```python
from build123d import *

# Parameters (mm, degrees)
F0_W      = 101.6
F0_H      = 63.5
F1_DEPTH  = 6.35
F2_W      = 101.6
F2_H      = 6.35
F3_DEPTH  = 6.35
F4_W      = 101.6
F4_H      = 20.32
F5_DEPTH  = 6.35
F6_W      = 101.6
F6_H      = 8.8265
F7_DEPTH  = 6.35
F8_W      = 12.7
F8_H      = 6.35
F9_DEPTH  = 6.35
F10_W     = 12.7
F10_H     = 6.35
F11_DEPTH = 6.35
F12_W     = 101.6
F12_H     = 6.9977
F13_DEPTH = 6.35
F14_W     = 12.7
F14_H     = 6.35
F15_DEPTH = 6.35
F16_W     = 12.7
F16_H     = 6.35
F17_DEPTH = 6.35
F19_DEPTH = 6.35


with BuildPart() as f1:
    # F0 (on Top) → F1 (new body)
    with BuildSketch(Plane.XY):
        Rectangle(F0_W, F0_H)
    extrude(amount=F1_DEPTH)

    # F2 (on face) → F3 (join)
    with BuildSketch(Plane.XY.offset(6.35)):
        with Locations((0, -28.575)):
            Rectangle(F2_W, F2_H)
    extrude(amount=F3_DEPTH)

    # F4 (on face) → F5 (join)
    with BuildSketch(Plane.XY.offset(6.35)):
        with Locations((0, 3.937)):
            Rectangle(F4_W, F4_H)
    extrude(amount=F5_DEPTH)

    # F6 (on face) → F7 (join)
    with BuildSketch(Plane.XY.offset(6.35)):
        with Locations((0, 27.33675)):
            Rectangle(F6_W, F6_H)
    extrude(amount=F7_DEPTH)

    # F8 (on face) → F9 (join)
    with BuildSketch(Plane.XZ.offset(31.75)):
        with Locations((-44.45, 3.175)):
            Rectangle(F8_W, F8_H)
        with Locations((-19.05, 3.175)):
            Rectangle(F8_W, F8_H)
        with Locations((6.35, 3.175)):
            Rectangle(F8_W, F8_H)
        with Locations((31.75, 3.175)):
            Rectangle(F8_W, F8_H)
    extrude(amount=F9_DEPTH)

    # F10 (on face) → F11 (join)
    with BuildSketch(Plane(origin=(0, 31.75, 0), x_dir=(-1, 0, 0), z_dir=(0, 1, 0))):
        with Locations((-44.45, 3.175)):
            Rectangle(F10_W, F10_H)
        with Locations((-19.05, 3.175)):
            Rectangle(F10_W, F10_H)
        with Locations((6.35, 3.175)):
            Rectangle(F10_W, F10_H)
        with Locations((31.75, 3.175)):
            Rectangle(F10_W, F10_H)
    extrude(amount=F11_DEPTH)

    # F12 (on face) → F13 (join)
    with BuildSketch(Plane.XY.offset(6.35)):
        with Locations((0, 19.42465)):
            Rectangle(F12_W, F12_H)
    extrude(amount=F13_DEPTH)

    # F14 (on face) → F15 (join)
    with BuildSketch(Plane.YZ.offset(50.8)):
        Polygon((-19.05, 0), (-19.05, 6.35), (-25.4, 6.35), (-31.75, 6.35), (-31.75, 0), align=None)
        Polygon((6.35, 6.35), (0, 6.35), (-6.223, 6.35), (-6.35, 6.35), (-6.35, 0), (6.35, 0), align=None)
        with Locations((25.4, 3.175)):
            Rectangle(F14_W, F14_H)
    extrude(amount=F15_DEPTH)

    # F16 (on face) → F17 (join)
    with BuildSketch(Plane(origin=(-50.8, 0, 0), x_dir=(0, -1, 0), z_dir=(-1, 0, 0))):
        with Locations((-25.4, 3.175)):
            Rectangle(F16_W, F16_H)
        Polygon((6.223, 6.35), (0, 6.35), (-6.35, 6.35), (-6.35, 0), (6.35, 0), (6.35, 6.35), align=None)
        Polygon((25.4, 6.35), (19.05, 6.35), (19.05, 0), (31.75, 0), (31.75, 6.35), align=None)
    extrude(amount=F17_DEPTH)

    # F18 (on face) → F19 (join)
    with BuildSketch(Plane.XY.offset(6.35)):
        Polygon((50.8, -6.223), (-50.8, -6.223), (-50.8, -6.35), (-50.8, -19.05), (50.8, -19.05), (50.8, -6.35), align=None)
    extrude(amount=F19_DEPTH)


solid = f1.part
```
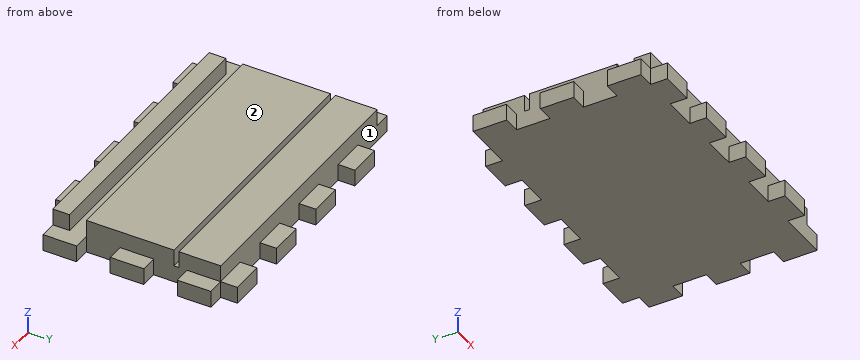
Can you work these out from the model? Positions are in its coordinate system, mm. Face numbers are marked on the shaded views. Round coordinates to 2 decimals unless told otherwise and drop trailing zeros. Loops run counter-clockwise (first coordinate to the right, second up) from the corner with the lowest first, then second, coordinate; pieces in that order, holes last. Notation, with made-up numbers: (72, 88) -> (96, 88) arc R15 cw to (96, 97) -> close; hole circle Ø1 at (-16.75, -32). An arc over 180 degrees is marked (long way). One line per item, written item: value. Start each with the question number.
1. If we section it at C-C, the plane x = -39.5: Write out the boundary of the cut face in (y, z).
2. If we mould it in two halves opening along X, with no side actions, what happens to the marked faces 1 and 2? For each: pulls with the +X half, pulls with the -X half, needs draft (parallel to the pull), parting line crosses it, or undercut.
3. If we section it at A-A, the plane z = 10.75: Write out the boundary of the cut face in (x, y), then the cut area to 3 significant figures.
4. If I drill on probe 1 along Y at (x, z) = (-2.5, 9.5); probe 2 along X at (y, z) = (7, 8.25); probe 3 along Y at (x, z) = (-9.5, 4.25), over which ranges is the centre line in solid material (lowest first)?
5. If we section it at B-B, the plane y = 5: Write out the boundary of the cut face in (x, z).
6. For pin 1 (3 mm diameter, centred on x = 14, z = 10.5, fed in from -Y); pin 2 (5 mm diameter, centred on y = -34.5, z = 1.5, fed in from +X); pin 3 (7 mm diameter, centred on y = -27.5, z = 10.5, fed in from -X), each with a flat end and sliding along its axis, tell me the tip position at first contact or that it passes through.
7. If we section it at D-D, the plane y = -23: Write out the boundary of the cut face in (x, z), then the cut area to 3 significant figures.
Calculated:
1. outline: (-38.1, 0) -> (31.75, 0) -> (31.75, 12.7) -> (15.93, 12.7) -> (15.93, 6.35) -> (14.1, 6.35) -> (14.1, 12.7) -> (-19.05, 12.7) -> (-19.05, 6.35) -> (-25.4, 6.35) -> (-25.4, 12.7) -> (-31.75, 12.7) -> (-31.75, 6.35) -> (-38.1, 6.35) -> close
2. face 1: undercut
2. face 2: needs draft
3. outline: (-50.8, -31.75) -> (50.8, -31.75) -> (50.8, -25.4) -> (-50.8, -25.4) -> close; (-50.8, -19.05) -> (50.8, -19.05) -> (50.8, 14.1) -> (-50.8, 14.1) -> close; (-50.8, 15.93) -> (50.8, 15.93) -> (50.8, 31.75) -> (-50.8, 31.75) -> close
3. area: 5,620 mm²
4. probe 1: y = -31.75 to -25.4, -19.05 to 14.1, 15.93 to 31.75
4. probe 2: x = -50.8 to 50.8
4. probe 3: y = -31.75 to 38.1
5. outline: (-57.15, 0) -> (57.15, 0) -> (57.15, 6.35) -> (50.8, 6.35) -> (50.8, 12.7) -> (-50.8, 12.7) -> (-50.8, 6.35) -> (-57.15, 6.35) -> close
6. pin 1: stops at y = -31.75
6. pin 2: stops at x = 38.1
6. pin 3: stops at x = -50.8
7. outline: (-57.15, 0) -> (57.15, 0) -> (57.15, 6.35) -> (-57.15, 6.35) -> close
7. area: 726 mm²
